```python
from build123d import *

# Parameters (mm, degrees)
SKETCH1_W                      = 15
SKETCH1_H                      = 35
BOSS_EXTRUDE1_DEPTH            = 20
SKETCH2_W                      = 15
SKETCH2_H                      = 10.2
CUT_EXTRUDE1_DEPTH             = 44.011626335
FILLET1_R                      = 2
SKETCH4_W                      = 13
SKETCH4_H                      = 14.8
CUT_EXTRUDE3_DEPTH             = 44.011626335
CUT_EXTRUDE4_REACH             = 45.012
SKETCH5_W                      = 5
SKETCH5_H                      = 9.8
CUT_EXTRUDE4_DIRECTION_2_DEPTH = 44.011626335
FILLET2_R                      = 2


with BuildPart() as part:
    # Sketch1 → Boss-Extrude1 (new body)
    with BuildSketch(Plane.XY):
        with Locations((-7.5, 17.5)):
            Rectangle(SKETCH1_W, SKETCH1_H)
    extrude(amount=BOSS_EXTRUDE1_DEPTH)

    # Sketch2 → Cut-Extrude1 (cut, through all)
    with BuildSketch(Plane(origin=(0, 0, 0), x_dir=(0, 0, -1), z_dir=(1, 0, 0))):
        with Locations((-12.5, 10.1)):
            Rectangle(SKETCH2_W, SKETCH2_H)
    extrude(amount=-CUT_EXTRUDE1_DEPTH, mode=Mode.SUBTRACT)

    # Fillet1
    fillet1_edges = [part.edges().sort_by_distance(p)[0] for p in [
        (-15, 15.2, 12.5),
        (-15, 10.1, 5),
        (-7.5, 15.2, 5),
        (-15, 5, 12.5),
        (-7.5, 5, 5),
        (0, 5, 12.5),
        (0, 10.1, 5),
        (0, 15.2, 12.5),
    ]]
    fillet(fillet1_edges, radius=FILLET1_R)

    # Sketch4 → Cut-Extrude3 (cut, through all)
    with BuildSketch(Plane.ZY.offset(15)):
        with Locations((13.5, 27.6)):
            Rectangle(SKETCH4_W, SKETCH4_H)
    extrude(amount=-CUT_EXTRUDE3_DEPTH, mode=Mode.SUBTRACT)

    # Sketch5 → Cut-Extrude4 (cut, up to next)
    with BuildSketch(Plane(origin=(0, 0, 0), x_dir=(-1, 0, 0), z_dir=(0, 0, -1)), mode=Mode.PRIVATE) as cut_extrude4_sk1:
        with Locations((7.5, 30.1)):
            Rectangle(SKETCH5_W, SKETCH5_H)
    cut_extrude4_tool1 = extrude(cut_extrude4_sk1.sketch, amount=-CUT_EXTRUDE4_REACH, mode=Mode.PRIVATE) & part.part
    add(cut_extrude4_tool1.solids().sort_by_distance((-7.5, 30.1, 0))[0], mode=Mode.SUBTRACT)

    # Sketch5 → Cut-Extrude4 direction 2 (cut)
    with BuildSketch(Plane(origin=(0, 0, 0), x_dir=(-1, 0, 0), z_dir=(0, 0, -1))):
        with Locations((7.5, 30.1)):
            Rectangle(SKETCH5_W, SKETCH5_H)
    extrude(amount=CUT_EXTRUDE4_DIRECTION_2_DEPTH, mode=Mode.SUBTRACT)

    # Fillet2
    fillet2_edges = [part.edges().sort_by_distance(p)[0] for p in [
        (-7.5, 0, 20),
        (-15, 1.5, 20),
        (-7.5, 5, 20),
        (-0.585786438, 4.414213562, 20),
        (-14.414213562, 4.414213562, 20),
        (0, 18.7, 20),
        (-7.5, 15.2, 20),
        (-0.585786438, 15.785786438, 20),
        (-14.414213562, 15.785786438, 20),
        (0, 1.5, 20),
        (-7.5, 0, 0),
        (-15, 17.5, 0),
        (-2.5, 35, 0),
        (0, 17.5, 0),
        (-15, 18.7, 20),
        (-15, 35, 3.5),
        (0, 35, 3.5),
        (0, 20.2, 13.5),
        (-7.5, 20.2, 20),
        (0, 27.6, 7),
        (-7.5, 20.2, 7),
        (-2.5, 35, 7),
        (-15, 27.6, 7),
        (-15, 20.2, 13.5),
        (-12.5, 35, 7),
        (0, 0, 10),
        (-15, 0, 10),
        (-12.5, 35, 0),
        (-5, 35, 3.5),
        (-5, 25.2, 3.5),
        (-10, 25.2, 3.5),
        (-10, 35, 3.5),
        (-5, 30.1, 0),
        (-7.5, 25.2, 0),
        (-10, 30.1, 0),
        (-7.5, 25.2, 7),
        (-5, 30.1, 7),
        (-10, 30.1, 7),
    ]]
    fillet(fillet2_edges, radius=FILLET2_R)


solid = part.part
```
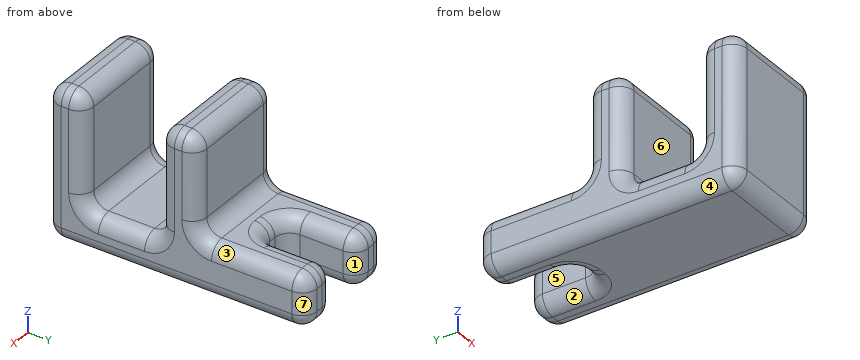
Here's how the part is built. I have some questions about the finished solid (model axes, mm). Face numbers are marked on the shaded views. A direction names the side the tool comes from. Coordinates: 2 decimals unless noted, no trailing zeros. Order: outer loops, then holes, each group sorted by start corner. A loop starts at its lowest first (then second) coordinate and runs counter-clockwise, first axis right, second up.
1) Imagine slicing it at C-C on y = 9.5. List the corners of the cut face in (x, z) for me.
2) Imagine slicing it at A-A on z = 16.5. List the corners of the cut face in (x, y) for me, and give its area (3 significant figures).
3) I need wall thicknesses on line 1 (Y direction, x = -9.25, z = 15.5); line 2 (Z direction, x = -4, y = 9); line 3 (Z direction, x = -2.5, y = 25.5). Which ranges of each line are inside material? Lowest first, please.
4) Will these pins go through, and if not, where does the flat tip stop? pin 1 (5 mm diameter, centred on x = -2, y = 16.5, fed in from +Z); pin 2 (2.5 mm diameter, centred on x = -5.5, z = 12, fed in from +Y); pin 3 (9 mm diameter, centred on x = -8.5, z = 12.5, fed in from +Y); pin 4 (1 mm diameter, centred on x = -4.5, y = 28, fed in from -Z).
5) Imagine slicing it at D-D on x = -1.25. List the corners of the cut face in (y, z) for me.
6) Which directions (+Z, -Z, +X, -X, +Y, -Y) give clear straight access to the entire face, cutting with the end or side of a thin tool? Please do the marked faces 1, 2 and 3.
7) We'd pull the mould along X, two halves only. Please class the marked faces 4, 5, 6 and 7: +X half, -X half, draft (parallel to the pull), parting line (faces both ways), or undercut.
8) Imagine slicing it at B-B on x = -12.5. List the corners of the cut face in (y, z) for me.
Response values:
1. outline: (-15, 2) arc R2 ccw to (-13, 0) - (-2, 0) arc R2 ccw to (0, 2) - (0, 3) arc R2 ccw to (-2, 5) - (-13, 5) arc R2 ccw to (-15, 3) - close
2. outline: (-15, 2) arc R2 ccw to (-13, 0) - (-2, 0) arc R2 ccw to (0, 2) - (0, 3) arc R2 ccw to (-2, 5) - (-13, 5) arc R2 ccw to (-15, 3) - close; (-15, 17.2) arc R2 ccw to (-13, 15.2) - (-2, 15.2) arc R2 ccw to (0, 17.2) - (0, 18.2) arc R2 ccw to (-2, 20.2) - (-13, 20.2) arc R2 ccw to (-15, 18.2) - close
2. area: 143 mm2
3. line 1: y = 0 to 5, 15.2 to 20.2
3. line 2: z = 0 to 5
3. line 3: z = 0 to 7
4. pin 1: stops at z = 20
4. pin 2: stops at y = 20.2
4. pin 3: stops at y = 20.47
4. pin 4: stops at z = 0.27
5. outline: (0.15, 2) arc R1.85 ccw to (2, 0.15) - (33, 0.15) arc R1.85 ccw to (34.85, 2) - (34.85, 5) arc R1.85 ccw to (33, 6.85) - (22.2, 6.85) arc R2.15 cw to (20.05, 9) - (20.05, 18) arc R1.85 ccw to (18.2, 19.85) - (17.2, 19.85) arc R1.85 ccw to (15.35, 18) - (15.35, 7) arc R2.15 cw to (13.2, 4.85) - (7, 4.85) arc R2.15 cw to (4.85, 7) - (4.85, 18) arc R1.85 ccw to (3, 19.85) - (2, 19.85) arc R1.85 ccw to (0.15, 18) - close
6. face 1: +Z, -Z, +Y
6. face 2: -Z, +Y
6. face 3: +Z, +X, +Y
7. face 4: -X half
7. face 5: undercut
7. face 6: draft
7. face 7: +X half
8. outline: (0, 2) arc R2 ccw to (2, 0) - (33, 0) arc R2 ccw to (35, 2) - (35, 5) arc R2 ccw to (33, 7) - (22.2, 7) arc R2 cw to (20.2, 9) - (20.2, 18) arc R2 ccw to (18.2, 20) - (17.2, 20) arc R2 ccw to (15.2, 18) - (15.2, 7) arc R2 cw to (13.2, 5) - (7, 5) arc R2 cw to (5, 7) - (5, 18) arc R2 ccw to (3, 20) - (2, 20) arc R2 ccw to (0, 18) - close
